```python
from build123d import *

# Parameters (mm, degrees)
SKETCH1_W                              = 300
SKETCH1_H                              = 150
BOSS_EXTRUDE1_DEPTH                    = 22
SKETCH2_R                              = 36
CUT_EXTRUDE1_DEPTH                     = 20
SKETCH3_R                              = 18.5
CUT_EXTRUDE2_DEPTH                     = 19
CBORE_FOR_M8_HEX_HEAD_BOLT1_AT_2_COUNT = 2
CBORE_FOR_M8_HEX_HEAD_BOLT1_AT_2_PITCH = 60
CBORE_FOR_M8_HEX_HEAD_BOLT1_AT_3_COUNT = 2
CBORE_FOR_M8_HEX_HEAD_BOLT1_AT_3_PITCH = 120
CIRPATTERN1_COUNT                      = 4


with BuildPart() as part:
    # Sketch1 → Boss-Extrude1 (new body)
    with BuildSketch(Plane.XY):
        Rectangle(SKETCH1_W, SKETCH1_H)
    extrude(amount=BOSS_EXTRUDE1_DEPTH)

    # Sketch2 → Cut-Extrude1 (cut)
    with BuildSketch(Plane.XY.offset(22)):
        with Locations((-60, 0)):
            Circle(SKETCH2_R)
    cut_extrude1 = extrude(amount=-CUT_EXTRUDE1_DEPTH, mode=Mode.SUBTRACT)

    # Sketch3 → Cut-Extrude2 (cut)
    with BuildSketch(Plane.XY.offset(2)):
        with Locations((-60, 0)):
            Circle(SKETCH3_R)
    cut_extrude2 = extrude(amount=-CUT_EXTRUDE2_DEPTH, mode=Mode.SUBTRACT)

    # Sketch6 → CBORE for M8 Hex Head Bolt1 (revolve, cut)
    with BuildSketch(Plane(origin=(-140, 60, 22), x_dir=(0, -1, 0), z_dir=(1, 0, 0))):
        Polygon((0, 0), (0, 27.5), (4.5, 24.796127214), (4.5, 5.3), (9.0055, 5.3), (9.0055, 0.025), (9.0305, 0), align=None)
    cbore_for_m8_hex_head_bolt1 = revolve(axis=Axis((-140, 60, 28.35), (0, 0, -1)), mode=Mode.SUBTRACT)

    # CBORE for M8 Hex Head Bolt1 at 2: CBORE for M8 Hex Head Bolt1 ×2
    with Locations(*[(0, -i * CBORE_FOR_M8_HEX_HEAD_BOLT1_AT_2_PITCH, 0) for i in range(1, CBORE_FOR_M8_HEX_HEAD_BOLT1_AT_2_COUNT)]):
        add(cbore_for_m8_hex_head_bolt1, mode=Mode.SUBTRACT)

    # CBORE for M8 Hex Head Bolt1 at 3: CBORE for M8 Hex Head Bolt1 ×2
    with Locations(*[(0, -i * CBORE_FOR_M8_HEX_HEAD_BOLT1_AT_3_PITCH, 0) for i in range(1, CBORE_FOR_M8_HEX_HEAD_BOLT1_AT_3_COUNT)]):
        add(cbore_for_m8_hex_head_bolt1, mode=Mode.SUBTRACT)

    # Mirror1: Cut-Extrude2, Cut-Extrude1, CBORE for M8 Hex Head Bolt1 across plane
    add(cut_extrude2.mirror(Plane(origin=(0, 0, 0), x_dir=(0, 0, 1), z_dir=(1, 0, 0))), mode=Mode.SUBTRACT)
    add(cut_extrude1.mirror(Plane(origin=(0, 0, 0), x_dir=(0, 0, 1), z_dir=(1, 0, 0))), mode=Mode.SUBTRACT)
    add(cbore_for_m8_hex_head_bolt1.mirror(Plane(origin=(0, 0, 0), x_dir=(0, 0, 1), z_dir=(1, 0, 0))), mode=Mode.SUBTRACT)

    # Mirror1 copy 1 sketch → Mirror1 copy 1 (revolve, cut)
    with BuildSketch(Plane(origin=(140, 0, 22), x_dir=(0, -1, 0), z_dir=(-1, 0, 0))):
        Polygon((0, 0), (0, -27.5), (4.5, -24.796127214), (4.5, -5.3), (9.0055, -5.3), (9.0055, -0.025), (9.0305, 0), align=None)
    revolve(axis=Axis((140, 0, 28.35), (0, 0, 1)), mode=Mode.SUBTRACT)

    # Mirror1 copy 2 sketch → Mirror1 copy 2 (revolve, cut)
    with BuildSketch(Plane(origin=(140, -60, 22), x_dir=(0, -1, 0), z_dir=(-1, 0, 0))):
        Polygon((0, 0), (0, -27.5), (4.5, -24.796127214), (4.5, -5.3), (9.0055, -5.3), (9.0055, -0.025), (9.0305, 0), align=None)
    revolve(axis=Axis((140, -60, 28.35), (0, 0, 1)), mode=Mode.SUBTRACT)

    # Sketch9 → Tap Drill for M6 Tap1 (revolve, cut)
    with BuildSketch(Plane(origin=(-29.9479618, 30.0520382, 22), x_dir=(0, -1, 0), z_dir=(1, 0, 0))):
        Polygon((0, 0), (0, 27.5), (2.5, 25.997848452), (2.5, 0.025), (2.525, 0), align=None)
    tap_drill_for_m6_tap1 = revolve(axis=Axis((-29.9479618, 30.0520382, 28.35), (0, 0, -1)), mode=Mode.SUBTRACT)

    # CirPattern1: Tap Drill for M6 Tap1 ×4 about axis
    cirpattern1_axis = Axis((-60, 0, 0), (0, 0, 1))
    for i in range(1, CIRPATTERN1_COUNT):
        add(tap_drill_for_m6_tap1.rotate(cirpattern1_axis, i * 360 / CIRPATTERN1_COUNT), mode=Mode.SUBTRACT)

    # Mirror2: Tap Drill for M6 Tap1 across plane
    add(tap_drill_for_m6_tap1.mirror(Plane(origin=(0, 0, 0), x_dir=(0, 0, 1), z_dir=(1, 0, 0))), mode=Mode.SUBTRACT)

    # Mirror2 copy 1 sketch → Mirror2 copy 1 (revolve, cut)
    with BuildSketch(Plane(origin=(90.0520382, 30.0520382, 22), x_dir=(-1, 0, 0), z_dir=(0, 1, 0))):
        Polygon((0, 0), (0, -27.5), (2.5, -25.997848452), (2.5, -0.025), (2.525, 0), align=None)
    revolve(axis=Axis((90.0520382, 30.0520382, 28.35), (0, 0, 1)), mode=Mode.SUBTRACT)

    # Mirror2 copy 2 sketch → Mirror2 copy 2 (revolve, cut)
    with BuildSketch(Plane(origin=(90.0520382, -30.0520382, 22), x_dir=(0, 1, 0), z_dir=(1, 0, 0))):
        Polygon((0, 0), (0, -27.5), (2.5, -25.997848452), (2.5, -0.025), (2.525, 0), align=None)
    revolve(axis=Axis((90.0520382, -30.0520382, 28.35), (0, 0, 1)), mode=Mode.SUBTRACT)

    # Mirror2 copy 3 sketch → Mirror2 copy 3 (revolve, cut)
    with BuildSketch(Plane(origin=(29.9479618, -30.0520382, 22), x_dir=(1, 0, 0), z_dir=(0, -1, 0))):
        Polygon((0, 0), (0, -27.5), (2.5, -25.997848452), (2.5, -0.025), (2.525, 0), align=None)
    revolve(axis=Axis((29.9479618, -30.0520382, 28.35), (0, 0, 1)), mode=Mode.SUBTRACT)


solid = part.part
```
Source: CAD feature listing. Evaluate the final solid. Frame: model axes, mm. A direction names the side the tool comes from. Round coordinates to 2 decimals unless told otherwise and drop trailing zeros. Loops run counter-clockwise (first coordinate to the right, second up) from the corner with the lowest first, then second, coordinate; pieces in that order, holes last.
(1) Section query A-A (x = 140). Give the number of separate pieces and of enclosed holes in the cut face, and give its area (3 significant figures).
From the geometry:
separate pieces: 4
enclosed holes: 0
area: 2,560 mm2
(2) Material intervals for probe 1 along X at (y, z) = (-60, 5); probe 2 along X at (y, z) = (60, 17.8); probe 3 along Y at (x, z) = (-60, 13.75), sorted ascending.
From the geometry:
probe 1: x = -150 to -144.5, -135.5 to 135.5, 144.5 to 150
probe 2: x = -150 to -149.01, -130.99 to 130.99, 149.01 to 150
probe 3: y = -75 to -36, 36 to 75
(3) Access query for faces 5 (the flat face through (-136, -56, 16.7)), 6 (the cylindrical face through (-78.482, 0.813, 1.014)). Directions: +Z, -Z, +X, -X, +Y, -Y. A direction counts if a zero-diameter tool reaches every point of the face in a straight line with its end or side. Return the directions, or none.
From the geometry:
face 5: +Z
face 6: +Z, -Z
(4) Section query C-C (x = 60). Output: boundary loops of the cut face in (y, z).
From the geometry:
outline: (-75, 0) - (-18.5, 0) - (-18.5, 2) - (-36, 2) - (-36, 22) - (-75, 22) - close; (18.5, 0) - (75, 0) - (75, 22) - (36, 22) - (36, 2) - (18.5, 2) - close
(5) Contact query for flat-ended pins moving along their axis: pin 1 Ø8 at (x, y) = (47, -15.5) entering from +Z; pin 2 Ø14.5 at (x, y) = (-140, 61.5) entering from +Z. Output: stop coordinate, or through.
From the geometry:
pin 1: stops at z = 2
pin 2: stops at z = 16.7
(6) Pull-direction query (Y, two-part tool) for faces 1 (the cylindrical face through (147.593, -64.841, 19.374)), 2 (the flat face through (-2, 75, 11)), 3 (the cylindrical face through (148.93, 1.17, 19.37)), 4 (the flat face through (-150, -1, 11)); classes: +Y half, -Y half, draft (parallel to the pull), parting line (faces both ways), or undercut.
From the geometry:
face 1: undercut
face 2: +Y half
face 3: undercut
face 4: draft
